Read the model definition and answer for the solid it produces. Units are mm, in the model's axes. A direction names the side the tool comes from. Coordinates: 2 decimals unless noted, no trailing zeros. Order: outer loops, then holes, each group sorted by start corner. A loop starts at its lowest first (then second) coordinate and runs counter-clockwise, first axis right, second up. Notation, with made-up numbers: (64, -17.5) - (119, -17.5) arc R12 cw to (119, -7.5) - close; hole circle Ø10 at (-29.5, 80.25). An arc over 180 degrees is marked (long way). Use one line per item in the form item = value.
```python
from build123d import *

# Parameters (mm, degrees)
F0_W     = 266.7
F0_H     = 127
F0_W_2   = 228.6
F0_H_2   = 12.7
F2_DEPTH = 6.35
F1_R     = 19.05
F3_DEPTH = 25.4
F4_W     = 267.121822
F4_H     = 123.204811
F5_DEPTH = 6.35


with BuildPart() as f2:
    # F0 (on Front) → F2 (new body)
    with BuildSketch(Plane.XZ):
        Rectangle(F0_W, F0_H)
        Polygon((114.3, -38.1), (114.3, -50.8), (-114.3, -50.8), (-114.3, -38.1), (-114.3, -25.4), (-114.3, -12.7), (-114.3, 0), (-114.3, 12.7), (-114.3, 25.4), (-114.3, 38.1), (-114.3, 50.8), (114.3, 50.8), (114.3, 38.1), (114.3, 25.4), (114.3, 12.7), (114.3, 0), (114.3, -12.7), (114.3, -25.4), align=None, mode=Mode.SUBTRACT)
        with Locations((0, -44.45)):
            Rectangle(F0_W_2, F0_H_2)
        with Locations((0, -31.75)):
            Rectangle(F0_W_2, F0_H_2)
        with Locations((0, -19.05)):
            Rectangle(F0_W_2, F0_H_2)
        with Locations((0, -6.35)):
            Rectangle(F0_W_2, F0_H_2)
        with Locations((0, 6.35)):
            Rectangle(F0_W_2, F0_H_2)
        with Locations((0, 19.05)):
            Rectangle(F0_W_2, F0_H_2)
        with Locations((0, 31.75)):
            Rectangle(F0_W_2, F0_H_2)
        with Locations((0, 44.45)):
            Rectangle(F0_W_2, F0_H_2)
    extrude(amount=F2_DEPTH)

    # F1 (on face) → F3 (join)
    with BuildSketch(Plane.XZ):
        with Locations((-133.560911, 63.970305)):
            Circle(F1_R)
        with Locations((133.389249, 63.660257)):
            Circle(F1_R)
        with Locations((133.079201, -63.458867)):
            Circle(F1_R)
        with Locations((-133.560911, -63.148819)):
            Circle(F1_R)
    extrude(amount=F3_DEPTH)

    # F4 (on face) → F5 (join)
    with BuildSketch(Plane(origin=(0, 0, 0), x_dir=(-1, 0, 0), z_dir=(0, 1, 0))):
        with Locations((0, -1.546413)):
            Rectangle(F4_W, F4_H)
    extrude(amount=F5_DEPTH)


solid = f2.part
```
(1) Section B-B, the plane z = 6 is taken. Write down the section's boundary in (x, y).
Answer list:
outline = (-133.56, 0) - (-133.35, 0) - (-133.35, -6.35) - (133.35, -6.35) - (133.35, 0) - (133.56, 0) - (133.56, 6.35) - (-133.56, 6.35) - close
(2) Section D-D, the plane z = -50.5 is taken. Write down the section's boundary in (x, y), then the cut area to 3 significant figures.
Answer list:
outline = (-147.81, -25.4) - (-119.32, -25.4) - (-119.32, -6.35) - (119.12, -6.35) - (119.12, -25.4) - (147.04, -25.4) - (147.04, 0) - (133.56, 0) - (133.56, 6.35) - (-133.56, 6.35) - (-133.56, 0) - (-147.81, 0) - close
area = 4,640 mm2
(3) Section A-A, the plane y = -3.5 is taken. Write down the section's boundary in (x, z).
Answer list:
outline = (-133.35, -44.1) arc R19.05 ccw (long way) to (-114.51, -63.5) - (114.03, -63.5) arc R19.05 ccw (long way) to (133.35, -44.41) - (133.35, 44.61) arc R19.05 ccw (long way) to (114.34, 63.5) - (-114.52, 63.5) arc R19.05 ccw (long way) to (-133.35, 44.92) - close
(4) Section C-C, the plane y = -16 is taken. Write down the section's boundary in (x, z).
Answer list:
outline = circle Ø38.1 at (-133.56, -63.15); circle Ø38.1 at (-133.56, 63.97); circle Ø38.1 at (133.08, -63.46); circle Ø38.1 at (133.39, 63.66)
(5) The mould has two halves that part along X. Classify faces 1 (the flat face through (133.561, 3, -2)), 2 (the flat face through (-2, -3, 63.5)), 3 (the flat face through (133, -25.4, -63)), 4 (the flat face through (-133.561, 3, -2)): +X half, -X half, draft (parallel to the pull), parting line (faces both ways), or undercut.
Answer list:
face_1 = +X half
face_2 = undercut
face_3 = draft
face_4 = -X half
(6) Which of the six approach directions +Z, -Z, +X, -X, +Y, -Y give full straight-line access (tool end or side, diameter ignored) to faces 5 (the flat face through (2, 3, -63.149)), 6 (the flat face through (-133.35, -3, 0)), 7 (the flat face through (133.35, -3, -1)), 8 (the cylindrical face through (-147.602, -12.522, 76.845))?
Answer list:
face_5 = -Z, +X, -X, +Y
face_6 = -X, -Y
face_7 = +X, -Y
face_8 = -Y
(7) Straight lines are drawn through the part: L1, parallel to Y at x = -116, z = -41; L2, parallel to X at y = -10, z = 62.5; L3, parallel to Z at x = 98.5, y = 3. For each, find the intervals that lie inside material, in ascending order.
Answer list:
L1 = -6.35 to 6.35
L2 = -152.55 to -114.57, 114.37 to 152.4
L3 = -63.15 to 60.06
(8) Given pin 1 Ø3 at (x, z) = (100.5, 34.5) entering from -Y; pin 2 Ø7 at (x, y) = (-11, -4) entering from -Z; pin 3 Ø5 at (x, y) = (9.5, 4.5) entering from +Z; pin 4 Ø5 at (y, z) = (-22, -39.5) entering from -X, each flat-ended and moving along its own axis, determine where each tip first touches the part or whether it passes through.
Answer list:
pin_1 = -6.35
pin_2 = -63.5
pin_3 = 60.06
pin_4 = through
